Source: three-view drawing plus pictorial views. Frame: mm from the lowest corner of the part. A direction names the side the tool comes from. Give positions to 0.01 mm unless a question says otherwise; leave off trailing zeros. Loops run counter-clockwise (first coordinate to the right, second up) from the corner with the lowest first, then second, coordinate; pieces in that order, holes last. Notation, with made-up numbers: (19, 58) -> (55, 58) arc R20 cw to (55, 95) -> close; hole circle Ø7 at (-23, -28.75). An arc over 180 degrees is marked (long way). Answer in a Markdown table with one row per item. Add a question column.
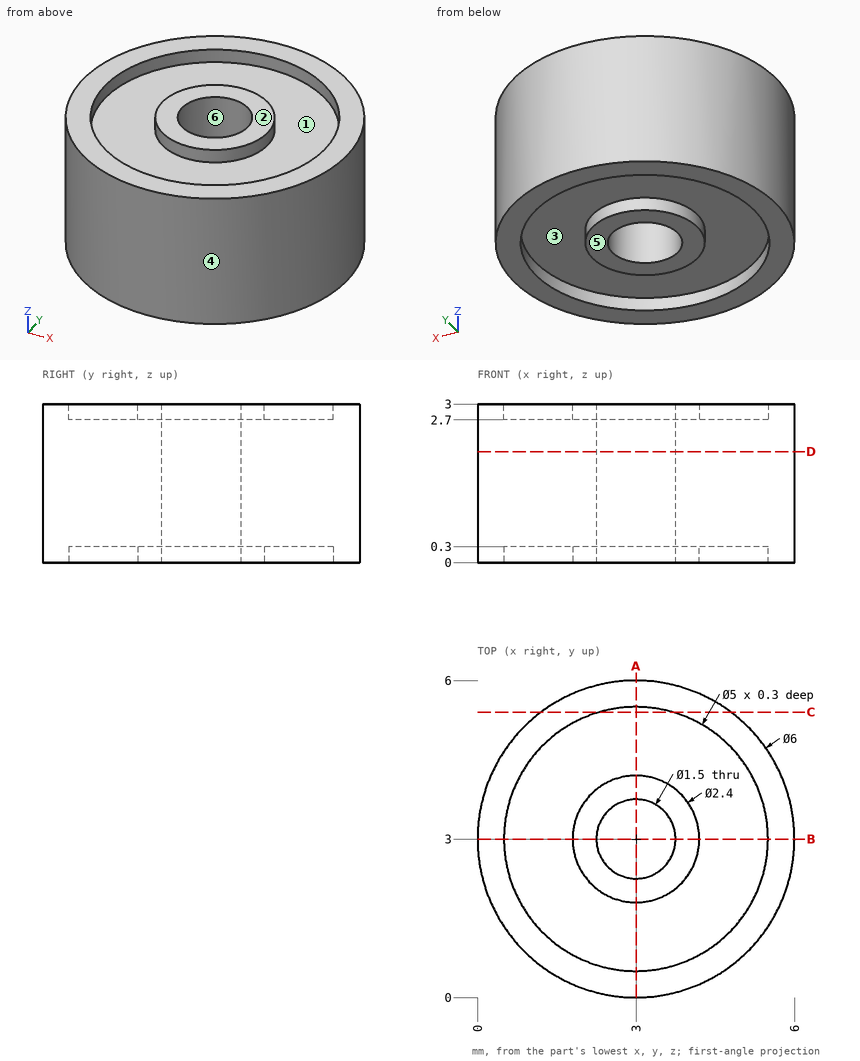
(1) Material intervals for line 1 along Y through (x, z) = (3, 2.9); line 2 along Y through (x, z) = (3, 2.3); line 3 along Y through (x, z) = (3.9, 0.2), sorted ascending. Write a range as from..to.
(2) Reachability of the marked faces 1, 2 and 3 from +Z, -Z, +X, -X, +Y, -Y: full face, straight path, thin tool, end or side. Return the list, or none.
(3) Pin query (flat end, axial travel): pin 1 Ø1.5 at (x, z) = (5.5, 1.5) entering from -Y. Return the tip coordinate at first contact, or that it passes through.
(4) Draft query along X for the marked faces 4, 5 and 6. Return one class per face: +X half, -X half, draft (parallel to the pull), parting line (faces both ways), or undercut.
(5) Cut plane D-D on z = 2.1. Return the cut outline in (x, y), then the cut area to 3 significant figures.
(6) Cut plane C-C on y = 5.4. Return the cut outline in (x, z), then the cut area to 3 significant figures.
(7) Cut plane A-A on x = 3. Return the cut outline in (y, z), then the cut area to 3 significant figures.
Answer list:
| question | item | result |
|---|---|---|
| 1 | line 1 | y = 0..0.5, 1.8..2.25, 3.75..4.2, 5.5..6 |
| 1 | line 2 | y = 0..2.25, 3.75..6 |
| 1 | line 3 | y = 0.14..0.67, 2.21..3.79, 5.33..5.86 |
| 2 | face 1 | +Z |
| 2 | face 2 | +Z, +X, -X, +Y, -Y |
| 2 | face 3 | -Z |
| 3 | pin 1 | stops at y = 0.56 |
| 4 | face 4 | parting line |
| 4 | face 5 | draft |
| 4 | face 6 | undercut |
| 5 | outline | circle Ø6 at (3, 3); hole circle Ø1.5 at (3, 3) |
| 5 | area | 26.5 mm² |
| 6 | outline | (1.2, 0) -> (2.3, 0) -> (2.3, 0.3) -> (3.7, 0.3) -> (3.7, 0) -> (4.8, 0) -> (4.8, 3) -> (3.7, 3) -> (3.7, 2.7) -> (2.3, 2.7) -> (2.3, 3) -> (1.2, 3) -> close |
| 6 | area | 9.96 mm² |
| 7 | outline | (0, 0) -> (0.5, 0) -> (0.5, 0.3) -> (1.8, 0.3) -> (1.8, 0) -> (2.25, 0) -> (2.25, 3) -> (1.8, 3) -> (1.8, 2.7) -> (0.5, 2.7) -> (0.5, 3) -> (0, 3) -> close; (3.75, 0) -> (4.2, 0) -> (4.2, 0.3) -> (5.5, 0.3) -> (5.5, 0) -> (6, 0) -> (6, 3) -> (5.5, 3) -> (5.5, 2.7) -> (4.2, 2.7) -> (4.2, 3) -> (3.75, 3) -> close |
| 7 | area | 11.9 mm² |
